from build123d import *

# Parameters (mm, degrees)
BOSS_EXTRUDE1_DEPTH = 5.35
BOSS_EXTRUDE3_DEPTH = 1
SKETCH4_R           = 3.555
BOSS_EXTRUDE4_DEPTH = 2.5
SKETCH5_R           = 1
CUT_EXTRUDE3_DEPTH  = 0.15
SKETCH3_R           = 2.5
CUT_EXTRUDE5_DEPTH  = 9.85


with BuildPart() as part:
    # Sketch2 → Boss-Extrude1 (new body)
    with BuildSketch(Plane(origin=(0, 0, 0), x_dir=(0, 0, -1), z_dir=(1, 0, 0))):
        Polygon((3.919437566, -2.29861752), (3.950379949, 2.245023741), (0.030942383, 4.54364126), (-3.919437566, 2.29861752), (-3.950379949, -2.245023741), (-0.030942383, -4.54364126), align=None)
    extrude(amount=BOSS_EXTRUDE1_DEPTH)

    # Sketch6 → Boss-Extrude3 (add)
    with BuildSketch(Plane.ZY):
        with BuildLine():
            Line((4.699218, 1.737080939), (4.210840713, 0.028675997))
            Line((4.210840713, 0.028675997), (4.722440239, -1.672919061))
            ThreePointArc((4.722440239, -1.672919061), (-5.009883831, -0.034117514), (4.699218, 1.737080939))
        make_face()
    extrude(amount=BOSS_EXTRUDE3_DEPTH)

    # Sketch4 → Boss-Extrude4 (add)
    with BuildSketch(Plane.ZY.offset(1)):
        Circle(SKETCH4_R)
    extrude(amount=BOSS_EXTRUDE4_DEPTH)

    # Sketch5 → Cut-Extrude3 (cut)
    with BuildSketch(Plane(origin=(0, 0.02679689, 3.934908757), x_dir=(1, 0, 0), z_dir=(0, -0.006809883, -0.999976812))):
        with Locations((2.675, 0)):
            Circle(SKETCH5_R)
    extrude(amount=CUT_EXTRUDE3_DEPTH, mode=Mode.SUBTRACT)

    # Sketch3 → Cut-Extrude5 (cut, through all)
    with BuildSketch(Plane.ZY.offset(3.5)):
        with Locations((0.79, 0)):
            Circle(SKETCH3_R)
    extrude(amount=-CUT_EXTRUDE5_DEPTH, mode=Mode.SUBTRACT)

    # Sketch7 → Cut-Revolve1 (revolve, cut)
    with BuildSketch(Plane.XY):
        Polygon((4.772649731, 4.54364126), (5.35, 3.54364126), (9.772649731, 3.54364126), (9.772649731, 8.54364126), (4.772649731, 8.54364126), align=None)
    revolve(axis=Axis((0, 0, 0), (1, 0, 0)), mode=Mode.SUBTRACT)


solid = part.part
Source: CAD feature listing. Evaluate the final solid. Frame: model axes, mm. A direction names the side the tool comes from. Round coordinates to 2 decimals unless told otherwise and drop trailing zeros. Loops run counter-clockwise (first coordinate to the right, second up) from the corner with the lowest first, then second, coordinate; pieces in that order, holes last. Notation, with made-up numbers: M -12.75,74 L 42.25,74 A11 cw 42.25,85 Z; hole C 60,-18 d11. An arc over 180 degrees is marked long. Return JSON: item names as keys, results as strings. Group by question number.
1. Section query A-A on x = 2.75. Output: boundary loops of the cut face in (y, z), and give its area (3 significant figures).
2. Pin query (flat end, axial travel): pin 1 (4 mm diameter, centred on x = -1, y = 2.5, fed in from -Z) (3 decimals); pin 2 (1.5 mm diameter, centred on x = -1.5, y = 2.5, fed in from +Z); pin 3 (4 mm diameter, centred on y = 0, z = 0.79, fed in from +X); pin 4 (1.5 mm diameter, centred on x = 2, z = -2.5, fed in from -Y). Return the tip coordinate at first contact, or that it passes through.
3. Mould query, pull axis Z, two halves, no side actions, for faces 1 (the face through (0.86, -2.44, 0.25)), 2 (the face through (0, -0.3, -4.1)), 3 (the face through (2.526, -3.437, -1.917)). Classes: released by +Z, released by -Z, zero draft, split by the parting line, or undercut.
4. Section query C-C on x = -1.5. Output: boundary loops of the cut face in (y, z) (3 decimals).
5. Material intervals for line 1 along X through (y, z) = (2.75, -3.75); line 2 along Y through (x, z) = (-2.75, -0.25); line 3 along Z through (x, y) = (-3, -1.5), sorted ascending. Write a range as from..to.
6. Section query B-B on x = 1.5. Output: boundary loops of the cut face in (y, z).
7. Reachability of faces 4 (the face through (-2.23, 1.07, 3.39)), 5 (the face through (-0.493, -0.81, 4.463)), 6 (the face through (2.526, 3.378, -2.018)), 7 (the face through (2.526, -3.378, 2.018)) from +Z, -Z, +X, -X, +Y, -Y: full face, straight path, thin tool, end or side. Return the list, or none.
Checks:
{
 "1": {"outline": "M -4.54,0.03 L -2.3,-3.92 L 2.25,-3.95 L 4.54,-0.03 L 2.3,3.92 L 1.02,3.93 L 1.02,3.78 L -0.97,3.79 L -0.97,3.94 L -2.25,3.95 Z; hole C 0,0.79 d5", "area": "33.7 mm²"},
 "2": {"pin 1": "stops at z = -4.985", "pin 2": "stops at z = 4.62", "pin 3": "passes through", "pin 4": "stops at y = -3.53"},
 "3": {"face 1": "undercut", "face 2": "zero draft", "face 3": "released by -Z"},
 "4": {"outline": "C 0,0 d7.11; hole C 0,0.79 d5"},
 "5": {"line 1": "x = -1..0", "line 2": "y = -3.55..-2.27, 2.27..3.55", "line 3": "z = -3.22..-1.21, 2.79..3.22"},
 "6": {"outline": "M -4.54,0.03 L -2.3,-3.92 L 2.25,-3.95 L 4.54,-0.03 L 2.3,3.92 L -2.25,3.95 Z; hole C 0,0.79 d5"},
 "7": {"face 4": "-X", "face 5": "+Z, +X, -X", "face 6": "-Z, +X, +Y", "face 7": "+Z, +X, -Y"}
}
